from build123d import *

# Parameters (mm, degrees)
SKETCH1_W           = 14
SKETCH1_H           = 6
BOSS_EXTRUDE1_DEPTH = 6
SKETCH2_W           = 5.4
SKETCH2_H           = 3.8
BOSS_EXTRUDE2_DEPTH = 4
CUT_EXTRUDE1_DEPTH  = 5.9


with BuildPart() as part:
    # Sketch1 → Boss-Extrude1 (new body)
    with BuildSketch(Plane(origin=(0, 0, 0), x_dir=(1, 0, 0), z_dir=(0, 1, 0))):
        Rectangle(SKETCH1_W, SKETCH1_H)
    extrude(amount=BOSS_EXTRUDE1_DEPTH)

    # Sketch2 → Boss-Extrude2 (add)
    with BuildSketch(Plane(origin=(0, 6, 0), x_dir=(1, 0, 0), z_dir=(0, 1, 0))):
        Rectangle(SKETCH2_W, SKETCH2_H)
    extrude(amount=BOSS_EXTRUDE2_DEPTH)

    # Sketch3 → Cut-Extrude1 (cut, through all)
    with BuildSketch(Plane.XY.offset(1.9)):
        with BuildLine():
            Line((-2.7, 10), (-2.7, 8.832137002))
            ThreePointArc((-2.7, 8.832137002), (-2.632889163, 9.008389319), (-2.465548082, 9.095370387))
            ThreePointArc((-2.465548082, 9.095370387), (-2.338024057, 9.145911014), (-2.252855325, 9.253442494))
            ThreePointArc((-2.252855325, 9.253442494), (-2.152197575, 9.371653244), (-2.002596083, 9.413188261))
            ThreePointArc((-2.002596083, 9.413188261), (-1.869202273, 9.445169874), (-1.769670652, 9.539563668))
            ThreePointArc((-1.769670652, 9.539563668), (-1.653294376, 9.642336847), (-1.499320058, 9.662278599))
            ThreePointArc((-1.499320058, 9.662278599), (-1.362742465, 9.67505722), (-1.250852111, 9.754412627))
            ThreePointArc((-1.250852111, 9.754412627), (-1.121100646, 9.839678807), (-0.96585391, 9.83762575))
            ThreePointArc((-0.96585391, 9.83762575), (-0.828842644, 9.83094407), (-0.706846566, 9.893663199))
            ThreePointArc((-0.706846566, 9.893663199), (-0.566332573, 9.959705471), (-0.412939448, 9.935698945))
            ThreePointArc((-0.412939448, 9.935698945), (-0.27825335, 9.909691506), (-0.148608047, 9.954511452))
            ThreePointArc((-0.148608047, 9.954511452), (-0.077790585, 9.98837122), (-0.000160897, 9.999999997))
            Line((-0.000160897, 10), (-2.7, 10))
        make_face()
        with BuildLine():
            Line((2.7, 10), (0.000160897, 10))
            ThreePointArc((0.000160897, 9.999999997), (0.077790585, 9.98837122), (0.148608047, 9.954511452))
            ThreePointArc((0.148608047, 9.954511452), (0.27825335, 9.909691506), (0.412939448, 9.935698945))
            ThreePointArc((0.412939448, 9.935698945), (0.566332573, 9.959705471), (0.706846566, 9.893663199))
            ThreePointArc((0.706846566, 9.893663199), (0.828842644, 9.83094407), (0.96585391, 9.83762575))
            ThreePointArc((0.96585391, 9.83762575), (1.121100646, 9.839678807), (1.250852111, 9.754412627))
            ThreePointArc((1.250852111, 9.754412627), (1.362742465, 9.67505722), (1.499320058, 9.662278599))
            ThreePointArc((1.499320058, 9.662278599), (1.653294376, 9.642336847), (1.769670652, 9.539563668))
            ThreePointArc((1.769670652, 9.539563668), (1.869202273, 9.445169874), (2.002596083, 9.413188261))
            ThreePointArc((2.002596083, 9.413188261), (2.152197575, 9.371653244), (2.252855325, 9.253442494))
            ThreePointArc((2.252855325, 9.253442494), (2.338024057, 9.145911014), (2.465548082, 9.095370387))
            ThreePointArc((2.465548082, 9.095370387), (2.632889163, 9.008389319), (2.7, 8.832137002))
            Line((2.7, 8.832137002), (2.7, 10))
        make_face()
    extrude(amount=-CUT_EXTRUDE1_DEPTH, mode=Mode.SUBTRACT)


solid = part.part
The model under review builds one solid part; all positions refer to its coordinate system, in mm. A direction names the side the tool comes from. Give positions to 0.01 mm unless a question says otherwise; leave off trailing zeros. Loops run counter-clockwise (first coordinate to the right, second up) from the corner with the lowest first, then second, coordinate; pieces in that order, holes last. Notation, with made-up numbers: (-1, 10) -> (25, 10) arc R12 cw to (25, 19) -> close; hole circle Ø6 at (15, 47.25). An arc over 180 degrees is marked (long way). Answer as a JSON object with one key per item and string values. Group by question number.
Q1. Tool access review of faces 1 (the flat face through (0, 8, 1.9)), 2 (the flat face through (2.7, 7, 0)), 3 (the flat face through (0, 8, -1.9)), 4 (the flat face through (-7, 3, 0)), 5 (the flat face through (-2.7, 7, 0)): name each direction out of +Z, -Z, +X, -X, +Y, -Y from which nothing blocks a thin tool from reaching the whole face with its end or side.
Q2. Take a section at B-B (y = 7.5). Write out the cut boundary in (x, z), plus the area to 3 significant figures.
Q3. Wall thickness on line 1 along Y through (x, z) = (3.5, -2.7); line 2 along Y through (x, z) = (1.5, -1.8); line 3 along Z through (x, y) = (0.75, 9): over which ranges is each line inside the solid? List them lowest first.
Q4. Take a section at A-A (x = -5.75). Write out the cut boundary in (y, z), plus the area to 3 significant figures.
Q5. Insertion check: pin 1 (4.5 mm diameter, centred on x = -0.5, y = 8, fed in from -Z); pin 2 (1 mm diameter, centred on x = -0.5, z = 2.5, fed in from +Y); pin 3 (2 mm diameter, centred on y = 8, z = -1.5, fed in from +X); pin 4 (2 mm diameter, centred on x = -1.5, z = 2, fed in from +Y). Each pin has a flat end and moves straight along its axis. Give the tip position at first contact, or say it passes through.
Answer below:
{
 "1": {"face 1": "+Z, +X, -X, +Y", "face 2": "+Z, -Z, +X, +Y", "face 3": "-Z, +X, -X, +Y", "face 4": "+Z, -Z, -X, +Y, -Y", "face 5": "+Z, -Z, -X, +Y"},
 "2": {"outline": "(-2.7, -1.9) -> (2.7, -1.9) -> (2.7, 1.9) -> (-2.7, 1.9) -> close", "area": "20.5 mm2"},
 "3": {"line 1": "y = 0 to 6", "line 2": "y = 0 to 9.66", "line 3": "z = -1.9 to 1.9"},
 "4": {"outline": "(0, -3) -> (6, -3) -> (6, 3) -> (0, 3) -> close", "area": "36.0 mm2"},
 "5": {"pin 1": "stops at z = -3", "pin 2": "stops at y = 6", "pin 3": "stops at x = 2.7", "pin 4": "stops at y = 9.96"}
}
